For this review, take the finished solid that the model builds, in its own axes (mm). A direction names the side the tool comes from. Give positions to 0.01 mm unless a question says otherwise; leave off trailing zeros. Loops run counter-clockwise (first coordinate to the right, second up) from the corner with the lowest first, then second, coordinate; pieces in that order, holes last. Notation, with made-up numbers: M 28.25,-22.75 L 34.25,-22.75 A13 cw 34.25,-8.75 Z; hole C -7,-11 d9. An arc over 180 degrees is marked long. Use CSV: the item, a comma, the result in double quotes. Start each with the question number.
1. To check wall thickness, follow line 1 (X direction, y = -12, z = 20); line 2 (X direction, y = 22.5, z = 2.5); line 3 (Y direction, x = 44.75, z = 2.55). State the ranges of each line that lie inside material, in increasing order. Write a range as [from, to].
2. The part is to be moulded in two halves that separate along Y. For faces 5 (the face through (-50, 0, 2)), 6 (the face through (41, 27, 2)), 7 (the face through (48.645, -25.572, 2.465)), 8 (the face through (-47.036, 20.881, 2.465)), say which applies: pulls with the +Y half, pulls with the -Y half, needs draft (parallel to the pull), parting line crosses it, or undercut.
3. Take a section at B-B, the plane z = 3.5. Write out the cut boundary in (x, y).
4. Tool access review of faces 1 (the face through (-41, 27, 2)), 2 (the face through (41, -27, 2)), 3 (the face through (40.25, 0, 15)), 4 (the face through (0, 24, 13)): name each direction out of +Z, -Z, +X, -X, +Y, -Y from which nothing blocks a thin tool from reaching the whole face with its end or side.
5. Take a section at D-D, the plane y = -17. Write out the cut boundary in (x, z), and give its area (3 significant figures).
6. Take a section at A-A, the plane x = -0.25. Write out the cut boundary in (y, z).
7. Insertion check: P1, Ø1.5, axis at x = -40, z = 2.5, coming from the +Y side; P2, Ø15, axis at x = 44.5, y = 6, coming from the +Z side; P3, Ø6, axis at x = 44.75, y = 22.25, coming from the +Z side; P4, Ø18, axis at x = -0.25, y = -7.75, coming from the +Z side. Each pin has a flat end and moves straight along its axis. Give the tip position at first contact, or say it passes through.
8. Take a section at C-C, the plane y = 16. Write out the cut boundary in (x, z).
from build123d import *

# Parameters (mm, degrees)
CROQUIS1_R              = 2.25
CROQUIS1_W              = 70.5
CROQUIS1_H              = 48
SALIENTE_EXTRUIR1_DEPTH = 5
CROQUIS1_3_W            = 80.5
CROQUIS1_3_H            = 2
CROQUIS1_3_H_2          = 54
CROQUIS1_3_W_2          = 70.5
CROQUIS1_3_H_3          = 48
SALIENTE_EXTRUIR2_DEPTH = 31
CROQUIS1_5_W            = 70.5
CROQUIS1_5_H            = 48
CORTAR_EXTRUIR2_DEPTH   = 27
REDONDEO4_R             = 5
REDONDEO5_START         = 5
REDONDEO5_DEPTH         = 26
REDONDEO5_START_2       = -1
REDONDEO5_2_DEPTH       = 8.65388
REDONDEO5_3_ANGLE       = 90
REDONDEO5_4_ANGLE       = 90
REDONDEO5_5_ANGLE       = 90
REDONDEO5_6_ANGLE       = 90
CROQUIS3_W              = 70.5
CROQUIS3_H              = 27
CORTAR_EXTRUIR5_DEPTH   = 80.183331618
CROQUIS4_R              = 11.399999943
CORTAR_EXTRUIR6_DEPTH   = 10


with BuildPart() as part:
    # Croquis1 → Saliente-Extruir1 (new body)
    with BuildSketch(Plane.XY):
        with BuildLine():
            Line((-45.25, 27), (45.25, 27))
            ThreePointArc((45.25, 27), (48.608757211, 25.608757211), (50, 22.25))
            Line((50, 22.25), (50, -22.25))
            ThreePointArc((50, -22.25), (48.608757211, -25.608757211), (45.25, -27))
            Line((45.25, -27), (-45.25, -27))
            ThreePointArc((-45.25, -27), (-48.608757211, -25.608757211), (-50, -22.25))
            Line((-50, -22.25), (-50, 22.25))
            ThreePointArc((-50, 22.25), (-48.608757211, 25.608757211), (-45.25, 27))
        make_face()
        with Locations((-45.25, 22.25)):
            Circle(CROQUIS1_R, mode=Mode.SUBTRACT)
        with Locations((44.75000048, 22.250001182)):
            Circle(CROQUIS1_R, mode=Mode.SUBTRACT)
        Rectangle(CROQUIS1_W, CROQUIS1_H, mode=Mode.SUBTRACT)
    extrude(amount=SALIENTE_EXTRUIR1_DEPTH)

    # Croquis1<3> → Saliente-Extruir2 (add)
    # profile 1 of 4: a face of its own
    with BuildSketch(Plane.XY):
        with Locations((0, 28)):
            Rectangle(CROQUIS1_3_W, CROQUIS1_3_H)
    # profile 2 of 4: a face of its own
    with BuildSketch(Plane.XY):
        Rectangle(CROQUIS1_3_W, CROQUIS1_3_H_2)
        Rectangle(CROQUIS1_3_W_2, CROQUIS1_3_H_3, mode=Mode.SUBTRACT)
    # profile 3 of 4: a face of its own
    with BuildSketch(Plane.XY):
        Rectangle(CROQUIS1_3_W_2, CROQUIS1_3_H_3)
    # profile 4 of 4: a face of its own
    with BuildSketch(Plane.XY):
        with Locations((0, -28)):
            Rectangle(CROQUIS1_3_W, CROQUIS1_3_H)
    extrude(amount=SALIENTE_EXTRUIR2_DEPTH)

    # Croquis1<5> → Cortar-Extruir2 (cut)
    with BuildSketch(Plane.XY):
        Rectangle(CROQUIS1_5_W, CROQUIS1_5_H)
    extrude(amount=CORTAR_EXTRUIR2_DEPTH, mode=Mode.SUBTRACT)

    # Redondeo4
    redondeo4_edges = [part.edges().sort_by_distance(p)[0] for p in [
        (40.25, 0, 31),
        (0, 29, 31),
        (-40.25, 0, 31),
        (0, -29, 31),
    ]]
    fillet(redondeo4_edges, radius=REDONDEO4_R)

    # Redondeo5: read off the stored shape, not the designer's step
    # Redondeo5 outline → Redondeo5 (cut)
    with BuildSketch(Plane.XY.offset(REDONDEO5_START)):
        with BuildLine():
            ThreePointArc((-40.25, 19), (-37.321067812, 26.071067812), (-30.25, 29))
            Line((-30.25, 29), (-40.25, 29))
            Line((-40.25, 29), (-40.25, 19))
        make_face()
        with BuildLine():
            Line((40.25, 29), (30.25, 29))
            ThreePointArc((30.25, 29), (37.321067812, 26.071067812), (40.25, 19))
            Line((40.25, 19), (40.25, 29))
        make_face()
        with BuildLine():
            Line((-40.25, -19), (-40.25, -29))
            Line((-40.25, -29), (-30.25, -29))
            ThreePointArc((-30.25, -29), (-37.321067812, -26.071067812), (-40.25, -19))
        make_face()
        with BuildLine():
            ThreePointArc((40.25, -19), (37.321067812, -26.071067812), (30.25, -29))
            Line((30.25, -29), (40.25, -29))
            Line((40.25, -29), (40.25, -19))
        make_face()
    extrude(amount=REDONDEO5_DEPTH, mode=Mode.SUBTRACT)

    # Redondeo5 2 outline → Redondeo5 2 (cut)
    with BuildSketch(Plane.XY.offset(REDONDEO5_START_2)):
        with BuildLine():
            Line((-40.25, 27), (-36.25, 27))
            ThreePointArc((-36.25, 27), (-33.41227766, 28.486832981), (-30.25, 29))
            Line((-30.25, 29), (-40.25, 29))
            Line((-40.25, 29), (-40.25, 27))
        make_face()
        with BuildLine():
            Line((40.25, 29), (30.25, 29))
            ThreePointArc((30.25, 29), (33.41227766, 28.486832981), (36.25, 27))
            Line((36.25, 27), (40.25, 27))
            Line((40.25, 27), (40.25, 29))
        make_face()
        with BuildLine():
            ThreePointArc((-30.25, -29), (-33.41227766, -28.486832981), (-36.25, -27))
            Line((-36.25, -27), (-40.25, -27))
            Line((-40.25, -27), (-40.25, -29))
            Line((-40.25, -29), (-30.25, -29))
        make_face()
        with BuildLine():
            ThreePointArc((36.25, -27), (33.41227766, -28.486832981), (30.25, -29))
            Line((30.25, -29), (40.25, -29))
            Line((40.25, -29), (40.25, -27))
            Line((40.25, -27), (36.25, -27))
        make_face()
    extrude(amount=REDONDEO5_2_DEPTH, mode=Mode.SUBTRACT)

    # Redondeo5 3 outline → Redondeo5 3 (revolve, cut)
    with BuildSketch(Plane(origin=(30.25, 19, 0), x_dir=(1, 0, 0), z_dir=(0, -1, 0))):
        with BuildLine():
            ThreePointArc((5, 31), (8.535533906, 29.535533906), (10, 26))
            Line((10, 26), (10, 31))
            Line((10, 31), (5, 31))
        make_face()
    revolve(axis=Axis((30.25, 19, 0), (0, 0, 1)), revolution_arc=REDONDEO5_3_ANGLE, mode=Mode.SUBTRACT)

    # Redondeo5 4 outline → Redondeo5 4 (revolve, cut)
    with BuildSketch(Plane(origin=(-30.25, 19, 0), x_dir=(0, 1, 0), z_dir=(1, 0, 0))):
        with BuildLine():
            ThreePointArc((5, 31), (8.535533906, 29.535533906), (10, 26))
            Line((10, 26), (10, 31))
            Line((10, 31), (5, 31))
        make_face()
    revolve(axis=Axis((-30.25, 19, 0), (0, 0, 1)), revolution_arc=REDONDEO5_4_ANGLE, mode=Mode.SUBTRACT)

    # Redondeo5 5 outline → Redondeo5 5 (revolve, cut)
    with BuildSketch(Plane(origin=(-30.25, -19, 0), x_dir=(-1, 0, 0), z_dir=(0, 1, 0))):
        with BuildLine():
            ThreePointArc((5, 31), (8.535533906, 29.535533906), (10, 26))
            Line((10, 26), (10, 31))
            Line((10, 31), (5, 31))
        make_face()
    revolve(axis=Axis((-30.25, -19, 0), (0, 0, 1)), revolution_arc=REDONDEO5_5_ANGLE, mode=Mode.SUBTRACT)

    # Redondeo5 6 outline → Redondeo5 6 (revolve, cut)
    with BuildSketch(Plane(origin=(30.25, -19, 0), x_dir=(0, -1, 0), z_dir=(-1, 0, 0))):
        with BuildLine():
            ThreePointArc((5, 31), (8.535533906, 29.535533906), (10, 26))
            Line((10, 26), (10, 31))
            Line((10, 31), (5, 31))
        make_face()
    revolve(axis=Axis((30.25, -19, 0), (0, 0, 1)), revolution_arc=REDONDEO5_6_ANGLE, mode=Mode.SUBTRACT)

    # Croquis3 → Cortar-Extruir5 (cut, through all)
    with BuildSketch(Plane(origin=(0, -24, 0), x_dir=(1, 0, 0), z_dir=(0, 1, 0))):
        with Locations((0, -13.5)):
            Rectangle(CROQUIS3_W, CROQUIS3_H)
    extrude(amount=-CORTAR_EXTRUIR5_DEPTH, mode=Mode.SUBTRACT)

    # Croquis4 → Cortar-Extruir6 (cut)
    with BuildSketch(Plane.XY.offset(31)):
        with Locations((-0.24999952, -7.749998818)):
            Circle(CROQUIS4_R)
    extrude(amount=-CORTAR_EXTRUIR6_DEPTH, mode=Mode.SUBTRACT)


solid = part.part
Result set:
1,line 1,"[-40.25, -35.25], [35.25, 40.25]"
1,line 2,"[-49.99, -47.49], [-43.01, -35.25], [35.25, 42.51], [46.99, 49.99]"
1,line 3,"[-27, 20], [24.5, 27]"
2,face 5,"needs draft"
2,face 6,"pulls with the +Y half"
2,face 7,"pulls with the -Y half"
2,face 8,"undercut"
3,outline,"M -50,-22.25 A4.75 ccw -45.25,-27 L -36.25,-27 A10 ccw -35.25,-27.66 L -35.25,24 L 35.25,24 L 35.25,-27.66 A10 ccw 36.25,-27 L 45.25,-27 A4.75 ccw 50,-22.25 L 50,22.25 A4.75 ccw 45.25,27 L 36.25,27 A10 ccw 30.25,29 L -30.25,29 A10 ccw -36.25,27 L -45.25,27 A4.75 ccw -50,22.25 Z; hole C -45.25,22.25 d4.5; hole C 44.75,22.25 d4.5"
4,face 1,"+Z, -Z, -X, +Y"
4,face 2,"+Z, -Z, +X, -Y"
4,face 3,"+Z, +X, +Y, -Y"
4,face 4,"-Z, -Y"
5,outline,"M -50,0 L -35.25,0 L -35.25,27 L -6.91,27 L -6.91,31 L -35.25,31 A5 ccw -40.25,26 L -40.25,5 L -50,5 Z; M 6.41,27 L 35.25,27 L 35.25,0 L 50,0 L 50,5 L 40.25,5 L 40.25,26 A5 ccw 35.25,31 L 6.41,31 Z"
5,area,"625 mm2"
6,outline,"M -28.9,27 L -19.15,27 L -19.15,31 L -24,31 A5 ccw Z; M 3.65,27 L 24,27 L 24,0 L 29,0 L 29,26 A5 ccw 24,31 L 3.65,31 Z"
7,P1,"y = 27"
7,P2,"z = 30.68"
7,P3,"z = 5"
7,P4,"through"
8,outline,"M -50,0 L -35.25,0 L -35.25,27 L 35.25,27 L 35.25,0 L 50,0 L 50,5 L 40.25,5 L 40.25,26 A5 ccw 35.25,31 L -35.25,31 A5 ccw -40.25,26 L -40.25,5 L -50,5 Z"
